Here's how the part is built. I have some questions about the finished solid (model axes, mm). A direction names the side the tool comes from. Round coordinates to 2 decimals unless told otherwise and drop trailing zeros. Order: outer loops, then holes, each group sorted by start corner. A loop starts at its lowest first (then second) coordinate and runs counter-clockwise, first axis right, second up. Notation, with made-up numbers: (-33, -8.5) - (-1, -8.5) arc R24 ccw to (-1, 19.5) - close; hole circle Ø1 at (76, 45.25). An arc over 180 degrees is marked (long way). Answer as a JSON object with one key per item and string values.
Autodesk Inventor part; units mm, degrees
ref_plane "YZ Plane" through (0, 0, 0) normal (1, 0, 0) x (0, 1, 0)
ref_plane "XZ Plane" through (0, 0, 0) normal (0, 1, 0) x (-1, 0, 0)
ref_plane "XY Plane" through (0, 0, 0) normal (0, 0, 1) x (1, 0, 0)
sketch "スケッチ1" plane through (0, 0, 0) normal (0, 0, 1) x (1, 0, 0)
  circle A0 centre (0, 0) radius 3
  dimension "d0" = 6
extrude "押し出し1" add sketch "スケッチ1" along normal blind 43
hole "穴1" at (0, 0, 0) direction (0, 0, 1) diameter 3 depth 6 tip angle 118
sketch "スケッチ2" plane through (0, 0, 43) normal (0, 0, 1) x (1, 0, 0)
  circle A0 centre (0, 0) radius 3
hole "穴2" at (0, 0, 43) direction (0, 0, -1) diameter 3 depth 6 tip angle 118
properties part number "スペーサ　m3-l42" material "アルミニウム 2014-T4"
1. If I drill on L1, parallel to Y at x = 0, z = 41.7; L2, parallel to Z at x = 0.9, y = 0.5; L3, parallel to Y at x = -1.35, z = 36.5, over which ranges is the centre line in solid material (lowest first)? Write a range as [from, to].
Responses:
{"L1": "[-3, -1.5], [1.5, 3]", "L2": "[6.28, 36.72]", "L3": "[-2.68, 2.68]"}
2. For faces 1 (the face through (1.3, -1.3, 0)), 2 (the face through (-0.07, 1.5, 39.96)), which set-ups out of +Z, -Z, +X, -X, +Y, -Y let a thin tool reach every point of the face, with its end or its side?
Responses:
{"face 1": "-Z, +X, -X, +Y, -Y", "face 2": "+Z"}
3. Imagine slicing it at B-B (x = 2.6). List the corners of the cut face in (y, z) for me.
Responses:
{"outline": "(-1.5, 0) - (1.5, 0) - (1.5, 43) - (-1.5, 43) - close"}
4. Thinking about a two-plate mould opening in Y: for faces 3 (the face through (1.3, -1.3, 43)), 4 (the face through (0.078, -0.248, 36.255)), 5 (the face through (-0.07, -1.5, 3.04)), 6 (the face through (-3, 0, 21)), which applies, pulls with the +Y half, pulls with the -Y half, needs draft (parallel to the pull), parting line crosses it, or undercut?
Responses:
{"face 3": "needs draft", "face 4": "undercut", "face 5": "undercut", "face 6": "parting line crosses it"}
5. For P1, Ø1, axis at x = 1, z = 35, coming from the +Y side; P2, Ø1.5, axis at y = 1, z = 8, coming from the +X side; P3, Ø1.8, axis at x = 0, y = 0, coming from the -Z side, each with a flat end and sliding along its axis, tell me the tip position at first contact or that it passes through.
Responses:
{"P1": "y = 2.96", "P2": "x = 2.99", "P3": "z = 6.36"}
6. Imagine slicing it at A-A (z = 35.5). List the corners of the cut face in (x, y) for me, plus the area to 3 significant figures.
Responses:
{"outline": "circle Ø6 at (0, 0)", "area": "28.3 mm2"}
7. Imagine slicing it at C-C (y = 1.9). List the corners of the cut face in (x, z) for me.
Responses:
{"outline": "(-2.32, 0) - (2.32, 0) - (2.32, 43) - (-2.32, 43) - close"}
